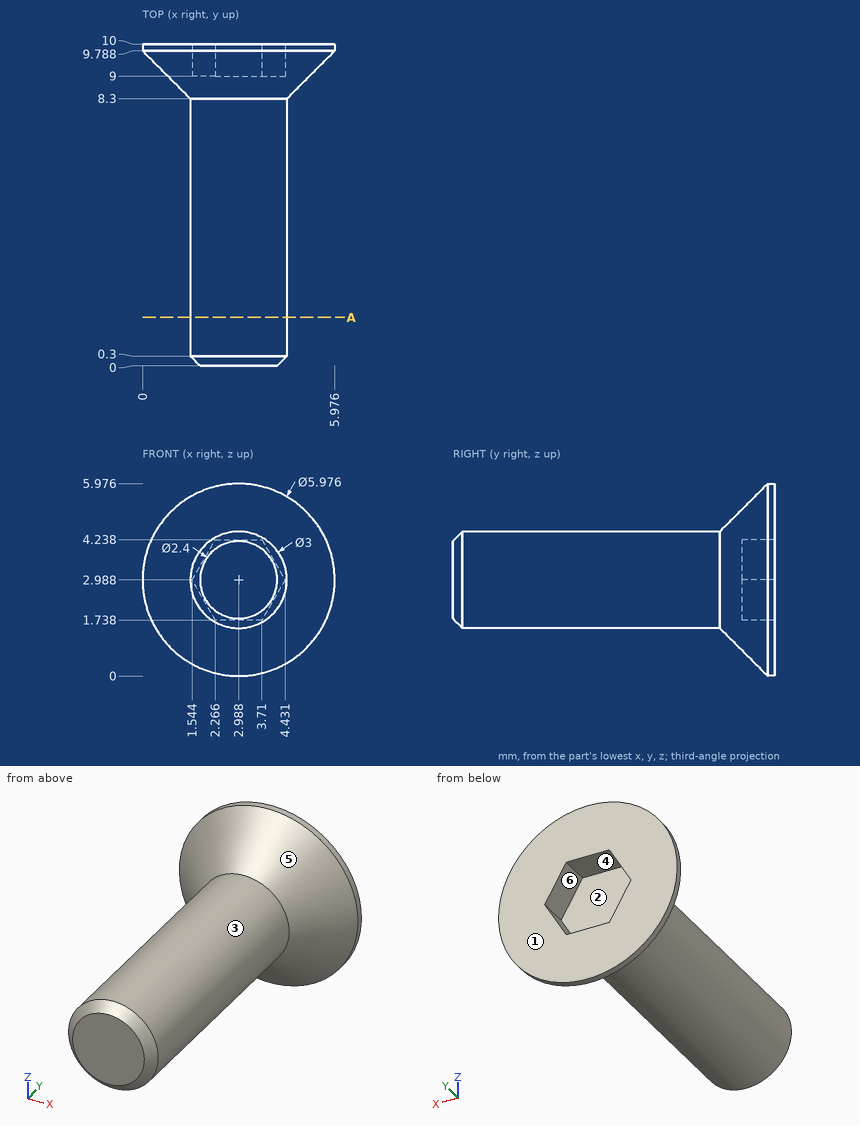
Check sheet for the drawn part. Datum: minimum x, y, z corner. Units: mm. A direction names the side the tool comes from. Give positions to 0.01 mm unless a question says otherwise; leave off trailing zeros. Order: outer loops, then holes, each group sorted by start corner. A loop starts at its lowest first (then second) coordinate and runs counter-clockwise, first axis right, second up.
1. Sectioned sample at A-A (y = 1.5). Record the boundary of the cut face in (x, z).
Completed:
outline: circle Ø3 at (2.99, 2.99)
2. Draft check along Z on the marked faces 1, 2, 3 and 4. Enter one of: pulls with the +Z half, pulls with the -Z half, needs draft (parallel to the pull), parting line crosses it, or undercut.
Completed:
face 1: needs draft
face 2: undercut
face 3: parting line crosses it
face 4: undercut
3. Depth check by flat-ended pin: pin 1 (0.8 mm diameter, centred on x = 2.5, y = 9.5, fed in from +Z); pin 2 (1 mm diameter, centred on x = 3.5, y = 6, fed in from -Z); pin 3 (0.7 mm diameter, centred on x = 2.5, z = 2.5, fed in from +Y). Enter the tip coordinate at first touch or a pass-through.
Completed:
pin 1: stops at z = 5.97
pin 2: stops at z = 1.49
pin 3: stops at y = 9
4. Access from +Z, -Z, +X, -X, +Y, -Y to the whole of each face (thin tool, end or side, straight path). Record for the marked faces 5 and 6.
Completed:
face 5: -Y
face 6: +Y
5. Scan lines: line 1 (X direction, y = 9.25, z = 1.05) (1 decimal); line 2 (Y direction, x = 3.05, z = 2.4); line 3 (Z direction, x = 5.3, y = 9.75) (1 decimal). Record each from-to range of solid material in increasing order.
Completed:
line 1: x = 1.5 to 4.5
line 2: y = 0 to 9
line 3: z = 1.2 to 4.8
